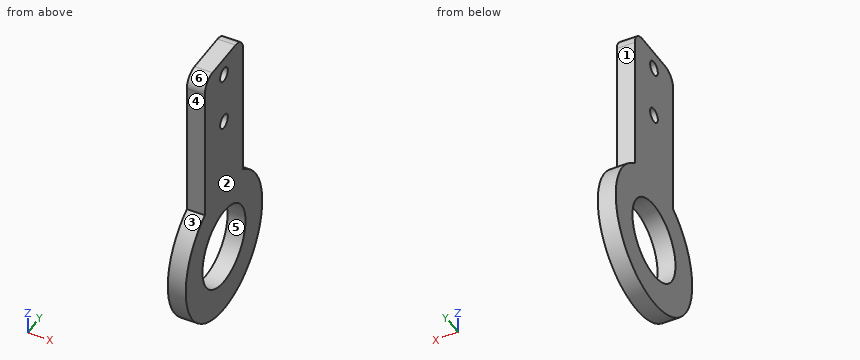
from build123d import *

# Parameters (mm, degrees)
SKETCH1_W              = 88.9
SKETCH1_H              = 25.4
BOSS_EXTRUDE1_DEPTH    = 3.175
FILLET1_R              = 12.7
F_10_CLEARANCE_HOLE1_D = 5.1054
FILLET2_R              = 5.08
SKETCH6_R              = 25.4
BOSS_EXTRUDE2_DEPTH    = 6.35
SKETCH7_R              = 14.2875
CUT_EXTRUDE1_DEPTH     = 63.861792847


with BuildPart() as part:
    # Sketch1 → Boss-Extrude1 (new, symmetric)
    with BuildSketch(Plane(origin=(0, 0, 0), x_dir=(0, 0, -1), z_dir=(1, 0, 0))):
        Rectangle(SKETCH1_W, SKETCH1_H)
    extrude(amount=BOSS_EXTRUDE1_DEPTH, both=True)

    # Fillet1
    fillet1_edges = [part.edges().sort_by_distance(p)[0] for p in [
        (0, -12.7, -44.45),
        (0, 12.7, -44.45),
    ]]
    fillet(fillet1_edges, radius=FILLET1_R - 0.0001)  # a hair under: the kernel refuses the full size

    # #10 Clearance Hole1 (through all)
    with Locations(Plane(origin=(3.175, 6.272913445, 168.827028559), x_dir=(0, 0, -1), z_dir=(1, 0, 0))):
        with Locations((149.777028559, -6.272913445), (130.727028559, -6.272913445)):
            Hole(F_10_CLEARANCE_HOLE1_D / 2)

    # Fillet2
    fillet2_edges = [part.edges().sort_by_distance(p)[0] for p in [
        (0, -12.7, 44.45),
        (0, 12.7, 44.45),
    ]]
    fillet(fillet2_edges, radius=FILLET2_R)

    # Sketch6 → Boss-Extrude2 (add)
    with BuildSketch(Plane(origin=(3.175, 0, 0), x_dir=(0, 0, -1), z_dir=(1, 0, 0))):
        with Locations((31.75, 0)):
            Circle(SKETCH6_R)
    extrude(amount=-BOSS_EXTRUDE2_DEPTH)

    # Sketch7 → Cut-Extrude1 (cut, through all)
    with BuildSketch(Plane(origin=(3.175, 0, 0), x_dir=(0, 0, -1), z_dir=(1, 0, 0))):
        with Locations((31.75, 0)):
            Circle(SKETCH7_R)
    extrude(amount=-CUT_EXTRUDE1_DEPTH, mode=Mode.SUBTRACT)


solid = part.part
The listing builds one solid part. Answer for the finished solid, in the listing's coordinates (mm). Face numbers are marked on the shaded views. A direction names the side the tool comes from. Coordinates: 2 decimals unless noted, no trailing zeros. Loops run counter-clockwise (first coordinate to the right, second up) from the corner with the lowest first, then second, coordinate; pieces in that order, holes last. Notation, with made-up numbers: (-24, 35.5) -> (27, 35.5) arc R25 ccw to (27, 61.5) -> close; hole circle Ø11 at (-26.75, 56.25). An arc over 180 degrees is marked (long way). Answer in a Markdown table with one row per item. Add a question column.
1. The part is cut by section B-B, the plane y = 0. Count the separate pieces of the cut face and the enclosed holes in it, then the cut area to 3 significant figures.
2. For the marked faces 1 and 2, determine the directions among +Z, -Z, +X, -X, +Y, -Y from which every point of the face is accessible in a straight line to the end or side of a thin tool.
3. The part is cut by section A-A, the plane z = -31.75. Write down the section's boundary in (x, y) (1 decimal), then the cut area to 3 significant figures.
4. Flat-ended cylindrical pins translate along their axes: P1, Ø4, axis at y = 0, z = 19.05, coming from the -X side; P2, Ø1.9, axis at x = 0, z = 21.5, coming from the -Y side; P3, Ø3, axis at x = -0.5, z = 5, coming from the +Y side. Find the tip coordinate at first contact, or state that the pin passes through.
5. Determine the mould class of the marked faces 3, 4, 5 and 6 for opening direction Z: +Z half, -Z half, draft (parallel to the pull), parting line (faces both ways), or undercut.
6. Consider line 1 (Y direction, x = -1.75, z = 10.5); line 2 (Y direction, x = 1.25, z = -31.75); line 3 (Z direction, x = 1.5, y = 11.5). Determine where each line is inside the solid, lowest interval first. Write a range as [from, to].
7. The part is cut by section C-C, the plane y = -6.5. Write down the section's boundary in (x, z) (3 decimals).
Answer below:
| question | item | result |
|---|---|---|
| 1 | separate pieces | 4 |
| 1 | enclosed holes | 0 |
| 1 | area | 399 mm2 |
| 2 | face 1 | +Z, +X, -X, +Y |
| 2 | face 2 | +Z, -Z, +X, +Y, -Y |
| 3 | outline | (-3.2, -25.4) -> (3.2, -25.4) -> (3.2, -14.3) -> (-3.2, -14.3) -> close; (-3.2, 14.3) -> (3.2, 14.3) -> (3.2, 25.4) -> (-3.2, 25.4) -> close |
| 3 | area | 141 mm2 |
| 4 | P1 | through |
| 4 | P2 | y = -12.7 |
| 4 | P3 | y = 12.7 |
| 5 | face 3 | parting line |
| 5 | face 4 | draft |
| 5 | face 5 | undercut |
| 5 | face 6 | +Z half |
| 6 | line 1 | [-12.7, 12.7] |
| 6 | line 2 | [-25.4, -14.29], [14.29, 25.4] |
| 6 | line 3 | [-54.4, -40.23], [-23.27, 42.65] |
| 7 | outline | (-3.175, -56.304) -> (3.175, -56.304) -> (3.175, -44.473) -> (-3.175, -44.473) -> close; (-3.175, -19.027) -> (3.175, -19.027) -> (3.175, 44.45) -> (-3.175, 44.45) -> close |
